Read the model definition and answer for the solid it produces. Units are mm, in the model's axes. Coordinates: 2 decimals unless noted, no trailing zeros. Loops run counter-clockwise (first coordinate to the right, second up) from the corner with the lowest first, then second, coordinate; pieces in that order, holes last. Notation, with made-up numbers: (-37, 15) - (-6, 15) arc R12 ccw to (-6, 28) - close; hole circle Ø7 at (23, -8). An arc over 180 degrees is marked (long way). Use CSV: the item, a comma, the result in double quotes.
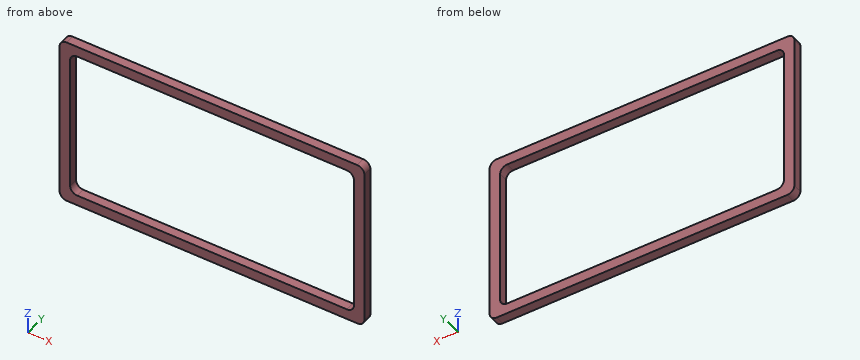
```python
from build123d import *

# Parameters (mm, degrees)
SKETCH1_W           = 66.8
SKETCH1_H           = 37.8
SKETCH1_W_2         = 62.2
SKETCH1_H_2         = 33.2
BOSS_EXTRUDE1_DEPTH = 2
FILLET1_R           = 1.55


with BuildPart() as part:
    # Sketch1 → Boss-Extrude1 (new body)
    with BuildSketch(Plane(origin=(0, 0, 0), x_dir=(1, 0, 0), z_dir=(0, 1, 0))):
        with Locations((33.4, 18.9)):
            Rectangle(SKETCH1_W, SKETCH1_H)
        with Locations((33.4, 18.9)):
            Rectangle(SKETCH1_W_2, SKETCH1_H_2, mode=Mode.SUBTRACT)
    extrude(amount=BOSS_EXTRUDE1_DEPTH)

    # Fillet1
    fillet1_edges = [part.edges().sort_by_distance(p)[0] for p in [
        (2.3, 1, -35.5),
        (2.3, 1, -2.3),
        (64.5, 1, -2.3),
        (64.5, 1, -35.5),
        (0, 1, -37.8),
        (66.8, 1, -37.8),
        (66.8, 1, 0),
        (0, 1, 0),
    ]]
    fillet(fillet1_edges, radius=FILLET1_R)


solid = part.part
```
Q1. The part is cut by section C-C on y = 0.6. Determine the outline of the cut face in (x, z).
Reported:
outline,"(0, -36.25) arc R1.55 ccw to (1.55, -37.8) - (65.25, -37.8) arc R1.55 ccw to (66.8, -36.25) - (66.8, -1.55) arc R1.55 ccw to (65.25, 0) - (1.55, 0) arc R1.55 ccw to (0, -1.55) - close; hole (2.3, -33.95) arc R1.55 ccw to (3.85, -35.5) - (62.95, -35.5) arc R1.55 ccw to (64.5, -33.95) - (64.5, -3.85) arc R1.55 ccw to (62.95, -2.3) - (3.85, -2.3) arc R1.55 ccw to (2.3, -3.85) - close"
Q2. Find the intervals of material crossed by probe 1 along Z at (x, y) = (23.5, 0.15); probe 2 along X at (y, z) = (0.4, -4); probe 3 along X at (y, z) = (1.7, -3), in increasing order. Write a range as [from, to].
Reported:
probe 1,"z = [-37.8, -35.5], [-2.3, 0]"
probe 2,"x = [0, 2.3], [64.5, 66.8]"
probe 3,"x = [0, 2.55], [64.25, 66.8]"
Q3. The part is cut by section A-A on x = 39.5. Determine the outline of the cut face in (y, z), and give its area (3 significant figures).
Reported:
outline,"(0, -37.8) - (2, -37.8) - (2, -35.5) - (0, -35.5) - close; (0, -2.3) - (2, -2.3) - (2, 0) - (0, 0) - close"
area,"9.20 mm²"
Q4. The part is cut by section B-B on z = -4.5. Determine the outline of the cut face in (x, y), and give its area (3 significant figures).
Reported:
outline,"(0, 0) - (2.3, 0) - (2.3, 2) - (0, 2) - close; (64.5, 0) - (66.8, 0) - (66.8, 2) - (64.5, 2) - close"
area,"9.20 mm²"
